Answer from the drawing. Dimensions are ordinates in mm from the lowest x, y and z of the part. Give positions to 0.01 mm unless a question says otherwise; leave off trailing zeros. Order: outer loops, then holes, each group sorted by start corner. A loop starts at its lowest first (then second) coordinate and runs counter-clockwise, first axis right, second up.
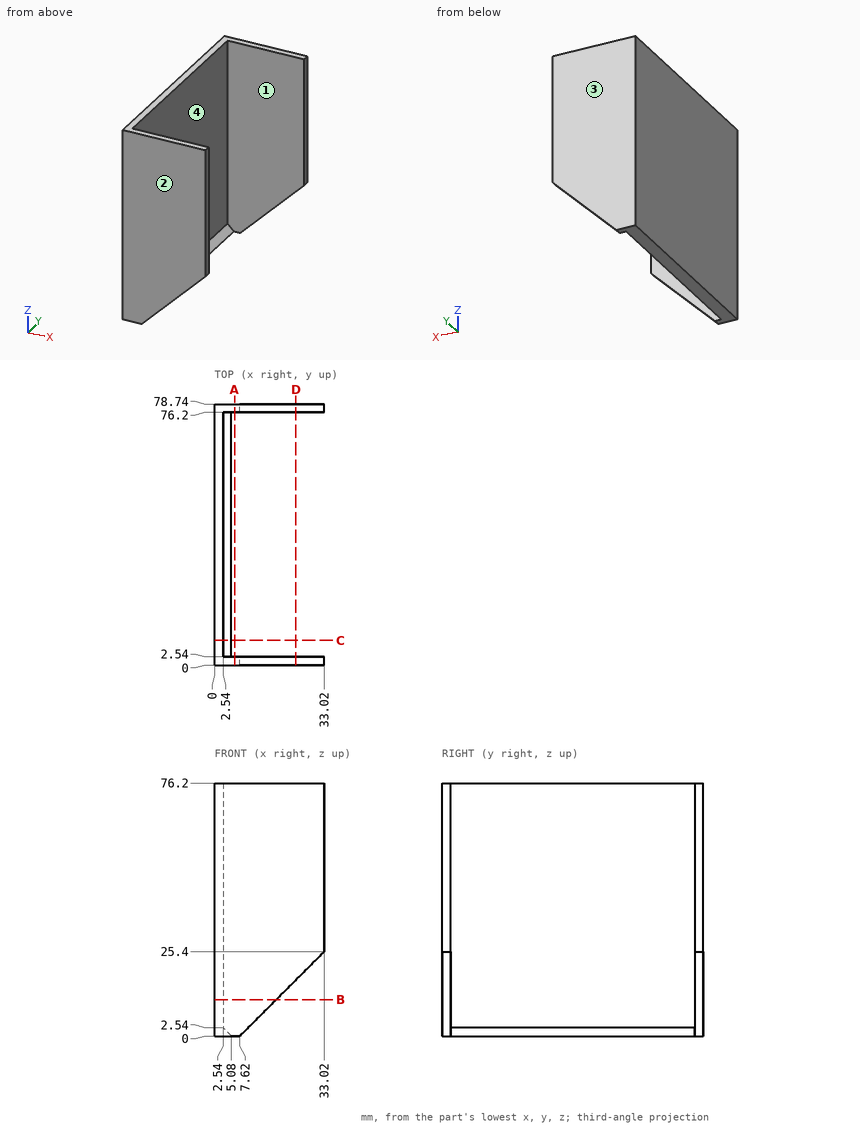
1. The part is cut by section A-A (x = 6). Write down the section's boundary in (y, z).
Findings below:
outline: (0, 0) - (2.54, 0) - (2.54, 76.2) - (0, 76.2) - close; (76.2, 0) - (78.74, 0) - (78.74, 76.2) - (76.2, 76.2) - close
2. The part is cut by section C-C (y = 7.5). Write down the section's boundary in (x, z), then the cut area to 3 significant figures.
Findings below:
outline: (0, 0) - (5.08, 0) - (2.54, 2.54) - (2.54, 76.2) - (0, 76.2) - close
area: 197 mm2
3. The part is cut by section B-B (z = 11). Write down the section's boundary in (x, y), then the cut area to 3 significant figures.
Findings below:
outline: (0, 0) - (18.62, 0) - (18.62, 2.54) - (2.54, 2.54) - (2.54, 76.2) - (18.62, 76.2) - (18.62, 78.74) - (0, 78.74) - close
area: 282 mm2
4. The part is cut by section D-D (x = 24.5). Write down the section's boundary in (y, z), then the cut area to 3 significant figures.
Findings below:
outline: (0, 16.88) - (2.54, 16.88) - (2.54, 76.2) - (0, 76.2) - close; (76.2, 16.88) - (78.74, 16.88) - (78.74, 76.2) - (76.2, 76.2) - close
area: 301 mm2
5. The mould has two halves that part along Y. Classify the marked faces 1, 2, 3 and 4: pulls with the +Y half, pulls with the -Y half, needs draft (parallel to the pull), parting line crosses it, or undercut.
Findings below:
face 1: undercut
face 2: pulls with the -Y half
face 3: pulls with the +Y half
face 4: undercut
6. Straight lines are drawn through the part: probe 1 along Y at (x, z) = (28, 26); probe 2 along X at (y, z) = (17.5, 13). For each, find the intervals that lie inside material, in ascending order.
Findings below:
probe 1: y = 0 to 2.54, 76.2 to 78.74
probe 2: x = 0 to 2.54
7. Given P1, Ø3, axis at y = 31, z = 41, coming from the +X side, flat-ended and moving along its own axis, determine where the tip first touches the part or whether it passes through.
Findings below:
P1: stops at x = 2.54
